The figure shows three views and two pictorial views of one solid part (mm, origin at its lowest corner). Answer the questions. A direction names the side the tool comes from. Coordinates: 2 decimals unless noted, no trailing zeros. Write each loop counter-clockwise with the first axis right and the second up, starting at its lowest first coordinate (ties: lowest second). Pieces come first, ordered by that corner, then holes. Notation, with made-up numbers: M -27,-1.75 L -4,-1.75 A16 cw -4,23.25 Z; hole C -34,-4 d7. An arc over 180 degrees is marked long. Write item = value, one per line.
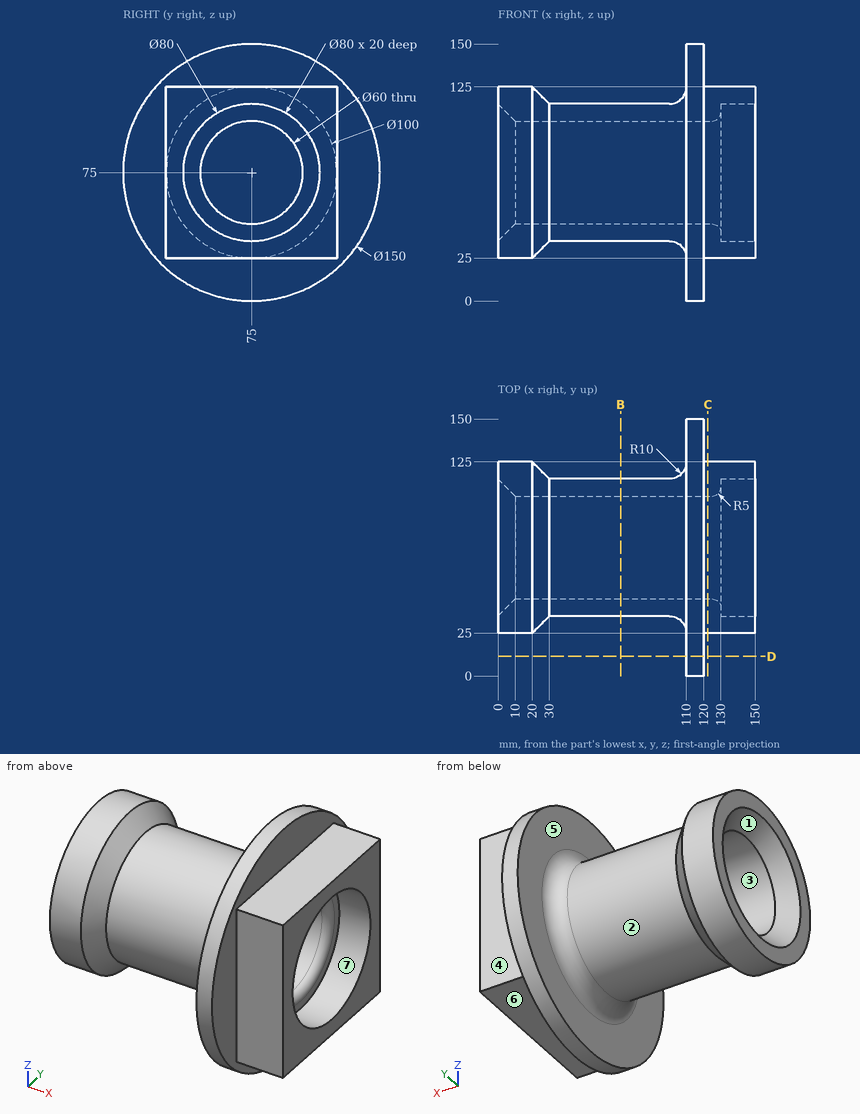
Item 1: Which of the six approach directions +Z, -Z, +X, -X, +Y, -Y give full straight-line access (tool end or side, diameter ignored) to the marked faces 4, 5, 6 and 7?
Worked answers:
face_4 = +Z, -Z, +X, +Y
face_5 = -X
face_6 = -Z, +X, +Y, -Y
face_7 = +X
Item 2: Find section D-D (y = 11.5). Determine the outline of the cut face in (x, z).
Worked answers:
outline = M 110,35.09 L 120,35.09 L 120,114.91 L 110,114.91 Z
Item 3: Flat-ended cylindrical pins translate along their axes: pin 1 (6 mm diameter, centred on x = 129, y = 62, fed in from -Z); pin 2 (15 mm diameter, centred on x = 137.5, y = 60.5, fed in from +Z); pin 3 (15 mm diameter, centred on x = 138, z = 93, fed in from -Y). Find the tip coordinate at first contact, or state that the pin passes through.
Worked answers:
pin_1 = 25
pin_2 = 125
pin_3 = 25
Item 4: Consider line 1 along Z through (x, y) = (137, 75); line 2 along Y through (x, z) = (120.5, 74.5); line 3 along X through (y, z) = (123.5, 128.5). Determine where each line is inside the solid, lowest interval first. Write a range as from..to.
Worked answers:
line_1 = 25..35, 115..125
line_2 = 25..45, 105..125
line_3 = 110..120
Item 5: Find section C-C (x = 122.5). Determine the outline of the cut face in (y, z), and give its area (3 significant figures).
Worked answers:
outline = M 25,25 L 125,25 L 125,125 L 25,125 Z; hole C 75,75 d60
area = 7,170 mm²
Item 6: For a pull along X with two mould halves and no side action, classify the marked faces 1, 2 and 3 as released by +X, released by -X, zero draft, split by the parting line, or undercut.
Worked answers:
face_1 = released by -X
face_2 = undercut
face_3 = zero draft
Item 7: Find section B-B (x = 71.5). Determine the outline of the cut face in (y, z), and give its area (3 significant figures).
Worked answers:
outline = C 75,75 d80; hole C 75,75 d60
area = 2,200 mm²
